```python
from build123d import *

# Parameters (mm, degrees)
SKETCH1_W                     = 15.500000000000002
SKETCH1_H                     = 20.5
BOSS_EXTRUDE1_DEPTH           = 2.35
BOSS_EXTRUDE1_TAPER           = 3.0000000000000067
BOSS_EXTRUDE1_OTHER_WAY_DEPTH = 2.35
BOSS_EXTRUDE1_OTHER_WAY_TAPER = 3.0000000000000067
SKETCH2_R                     = 1.9300000000000004
CUT_EXTRUDE1_DEPTH            = 14.682653417374864
SKETCH3_R                     = 2.7499999999999982
CUT_EXTRUDE2_DEPTH            = 3.2
CUT_EXTRUDE2_DRAFT            = -4.000000000000009
SKETCH3_R_2                   = 2.75
CUT_EXTRUDE2_PROFILE_2_DEPTH  = 3.2
CUT_EXTRUDE2_PROFILE_2_DRAFT  = -4.000000000000009
SKETCH4_R                     = 3.305
CUT_EXTRUDE3_DEPTH            = 0.001
BOSS_EXTRUDE2_DEPTH           = 0.61
CHAMFER1_SIZE                 = 0.3


with BuildPart() as part:
    # Sketch1 → Boss-Extrude1 (new body)
    with BuildSketch(Plane.XY):
        Rectangle(SKETCH1_W, SKETCH1_H)
    extrude(amount=BOSS_EXTRUDE1_DEPTH, taper=BOSS_EXTRUDE1_TAPER)

    # Sketch1 → Boss-Extrude1 other way (add)
    with BuildSketch(Plane.XY):
        Rectangle(SKETCH1_W, SKETCH1_H)
    extrude(amount=-BOSS_EXTRUDE1_OTHER_WAY_DEPTH, taper=BOSS_EXTRUDE1_OTHER_WAY_TAPER)

    # Sketch2 → Cut-Extrude1 (cut, through all)
    with BuildSketch(Plane.XY.offset(2.35)):
        with Locations((0, 4.790000000000001)):
            Circle(SKETCH2_R)
    extrude(amount=-CUT_EXTRUDE1_DEPTH, mode=Mode.SUBTRACT)


with BuildPart() as cut_extrude2_tool:
    # Sketch3 → Cut-Extrude2 (with draft: the straight prism first)
    with BuildSketch(Plane.XY.offset(2.35)):
        with Locations((7.75, 4.790000000000001)):
            Circle(SKETCH3_R)
    extrude(amount=-CUT_EXTRUDE2_DEPTH)
    # Cut-Extrude2: the draft: its side faces are tilted about the plane it starts from
    cut_extrude2_sides = [cut_extrude2_tool.faces().sort_by_distance(p)[0] for p in [
        (5, 4.79, 0.75),
    ]]
    draft(cut_extrude2_sides, Plane.XY.offset(2.35), CUT_EXTRUDE2_DRAFT)


with BuildPart() as part_1:
    add(part.part)

    # Cut-Extrude2: cut by cut_extrude2_tool
    add(cut_extrude2_tool.part, mode=Mode.SUBTRACT)


with BuildPart() as cut_extrude2_profile_2_tool:
    # Sketch3 → Cut-Extrude2 profile 2 (with draft: the straight prism first)
    with BuildSketch(Plane.XY.offset(2.35)):
        with Locations((-7.75, 4.790000000000001)):
            Circle(SKETCH3_R_2)
    extrude(amount=-CUT_EXTRUDE2_PROFILE_2_DEPTH)
    # Cut-Extrude2 profile 2: the draft: its side faces are tilted about the plane it starts from
    cut_extrude2_profile_2_sides = [cut_extrude2_profile_2_tool.faces().sort_by_distance(p)[0] for p in [
        (-10.5, 4.79, 0.75),
    ]]
    draft(cut_extrude2_profile_2_sides, Plane.XY.offset(2.35), CUT_EXTRUDE2_PROFILE_2_DRAFT)


with BuildPart() as part_2:
    add(part_1.part)

    # Cut-Extrude2 profile 2: cut by cut_extrude2_profile_2_tool
    add(cut_extrude2_profile_2_tool.part, mode=Mode.SUBTRACT)

    # Sketch4 → Cut-Extrude3 (cut)
    with BuildSketch(Plane(origin=(0, 0, -2.35), x_dir=(-1, 0, 0), z_dir=(0, 0, -1))):
        Polygon((-6.539115869693152, 8.755028571929065), (-5.095312145144818, 9.74), (-3.520299832613913, 9.74), (-3.520299832613913, 9.540000000000001), (3.520299832613913, 9.540000000000001), (3.520299832613913, 9.74), (4.827080405758514, 9.74), (6.2708841303068485, 8.755028571929065), (6.270884130306849, 1.9970301626645939), (6.07088413030685, 1.9970301626645939), (6.070884130306851, -3.3399999999999994), (-6.339115869693153, -3.3400000000000007), (-6.339115869693152, 1.9970301626645925), (-6.539115869693152, 1.997030162664592), align=None)
        with Locations((0, 4.790000000000001)):
            Circle(SKETCH4_R, mode=Mode.SUBTRACT)
    extrude(amount=-CUT_EXTRUDE3_DEPTH, mode=Mode.SUBTRACT)

    # Sketch6 → Boss-Extrude2 (add)
    with BuildSketch(Plane(origin=(0, 0, 0.14999999999999997), x_dir=(-1, 0, 0), z_dir=(0, 0, -1))):
        Polygon((-6.1850000000000005, -10.126841718684854), (-6.184999999999995, -30.249999999999993), (-4.934999999999998, -30.249999999999993), (-4.934999999999998, -14.049999999999999), (-4.484999999999999, -14.049999999999999), (-4.485, -10.126841718684854), align=None)
        Polygon((4.485000000000002, -10.126841718684853), (6.185000000000002, -10.126841718684853), (6.185000000000002, -30.249999999999993), (4.935000000000004, -30.249999999999993), (4.935000000000001, -14.049999999999997), (4.485000000000003, -14.049999999999997), align=None)
        Polygon((-1.3099999999999987, -10.126841718684854), (1.3100000000000005, -10.126841718684854), (1.3100000000000016, -14.05), (0.6250000000000014, -14.05), (0.6250000000000027, -30.249999999999993), (-0.624999999999995, -30.249999999999993), (-0.6249999999999972, -14.049999999999999), (-1.3099999999999983, -14.049999999999999), align=None)
    extrude(amount=BOSS_EXTRUDE2_DEPTH)

    # Chamfer1
    chamfer1_edges = [part_2.edges().sort_by_distance(p)[0] for p in [
        (6.184999999999995, -30.249999999999993, -0.15500000000000003),
        (4.934999999999998, -30.249999999999993, -0.15500000000000003),
        (-4.935000000000004, -30.249999999999993, -0.15500000000000003),
        (-6.185000000000002, -30.249999999999993, -0.15500000000000003),
        (0.624999999999995, -30.249999999999993, -0.15500000000000003),
        (-0.6250000000000027, -30.249999999999993, -0.15500000000000003),
    ]]
    chamfer(chamfer1_edges, length=CHAMFER1_SIZE)


solid = part_2.part
```
The model under review builds one solid part; all positions refer to its coordinate system, in mm. A direction names the side the tool comes from. Round coordinates to 2 decimals unless told otherwise and drop trailing zeros. Write each loop counter-clockwise with the first axis right and the second up, starting at its lowest first coordinate (ties: lowest second). Pieces come first, ordered by that corner, then holes. Notation, with made-up numbers: M 56.5,-22 L 83.5,-22 A13 ccw 83.5,-3 Z; hole C 44,34.5 d9. An arc over 180 degrees is marked long. Use CSV: the item, a comma, the result in double quotes. Start each with the question number.
(1) We need section A-A, the plane y = -14.5. State the section outline as (x, z) points (3 decimals).
(2) We need section B-B, the plane z = 1.95. State the section outline as (x, y) points, then the cut area to 3 significant figures.
(3) The part is to be moulded in two halves that separate along Y. For faces 4 (the face through (-0.11, 10.19, 1.16)), 5 (the face through (-5.11, 4.73, 0.77)), 6 (the face through (-7, 5, -0.85)), 7 (the face through (6, -20, 0.15)), say which applies: +Y half, -Y half, draft (parallel to the pull), parting line (faces both ways), or undercut.
(4) Clearance check with flat-ended pins moving along their axes: P1, Ø1.4, axis at x = 5.5, y = -19, coming from the -Z side; P2, Ø0.5, axis at y = -12.5, z = 0, coming from the -X side (3 decimals); P3, Ø0.5, axis at y = -21, z = -0.5, coming from the +X side (3 decimals). State where each tip first meets the part, or that it passes through.
(5) For line 1 along X through (y, z) = (-11, 0) (3 decimals); line 2 along Z through (x, y) = (4.25, -1); line 3 along Y through (x, z) = (0, -0.6), list the stretches that pass through material, from the lowest coordinate up.
(6) Tool access review of faces 1 (the face through (-6, -20, -0.46)), 2 (the face through (0, -18, 0.15)), 3 (the face through (7, 5, -0.85)): name each direction out of +Z, -Z, +X, -X, +Y, -Y from which nothing blocks a thin tool from reaching the whole face with its end or side.
Findings:
1,outline,"M -6.185,-0.46 L -4.935,-0.46 L -4.935,0.15 L -6.185,0.15 Z; M -0.625,-0.46 L 0.625,-0.46 L 0.625,0.15 L -0.625,0.15 Z; M 4.935,-0.46 L 6.185,-0.46 L 6.185,0.15 L 4.935,0.15 Z"
2,outline,"M -7.65,-10.15 L 7.65,-10.15 L 7.65,2.07 A2.72 cw 7.65,7.51 L 7.65,10.15 L -7.65,10.15 L -7.65,7.51 A2.72 cw -7.65,2.07 Z; hole C 0,4.79 d3.86"
2,area,"277 mm^2"
3,face 4,"+Y half"
3,face 5,"undercut"
3,face 6,"undercut"
3,face 7,"draft"
4,P1,"z = -0.46"
4,P2,"x = -6.185"
4,P3,"x = 6.185"
5,line 1,"-6.185 to -4.485, -1.31 to 1.31, 4.485 to 6.185"
5,line 2,"-2.35 to 2.35"
5,line 3,"-10.22 to 2.86, 6.72 to 10.22"
6,face 1,"-Z, +X, -X, -Y"
6,face 2,"+Z, +X, -X, -Y"
6,face 3,"+Z, +X"
